Verification items for this drawing (mm, ordinates from the low corner). Round coordinates to 2 decimals unless told otherwise and drop trailing zeros. Order: outer loops, then holes, each group sorted by start corner. A loop starts at its lowest first (then second) coordinate and runs counter-clockwise, first axis right, second up. Notation, with made-up numbers: M -30.5,22.5 L -19.5,22.5 A12 ccw -19.5,30.5 Z; hole C 58.5,12.5 d5. An arc over 180 degrees is marked long. Use CSV: the item, a comma, the result in double quotes. Start each with the question number.
Q1. Sectioned sample at D-D (y = 6.5). Enter the section's corners in (x, z), and give its area (3 significant figures).
Q2. Scan lines: line 1 (Y direction, x = 20, z = 2.1); line 2 (Y direction, x = 20, z = 4.5); line 3 (X direction, y = 31.5, z = 0.9). Record each from-to range of solid material in increasing order.
Q3. Sectioned sample at C-C (z = 1.15). Enter the section's corners in (x, y).
Q4. Gauge pin test, flat ends, axial feed: pin 1 Ø0.9 at (x, y) = (45.5, 45) entering from +Z; pin 2 Ø2.5 at (x, y) = (20, 45) entering from +Z; pin 3 Ø3 at (x, z) = (29, 1.5) entering from +Y. Record the tip position at first contact, or that the pin passes through.
Q5. Sectioned sample at A-A (x = 45). Enter the section's corners in (y, z).
Q6. Sectioned sample at B-B (y = 45). Enter the section's corners in (x, z).
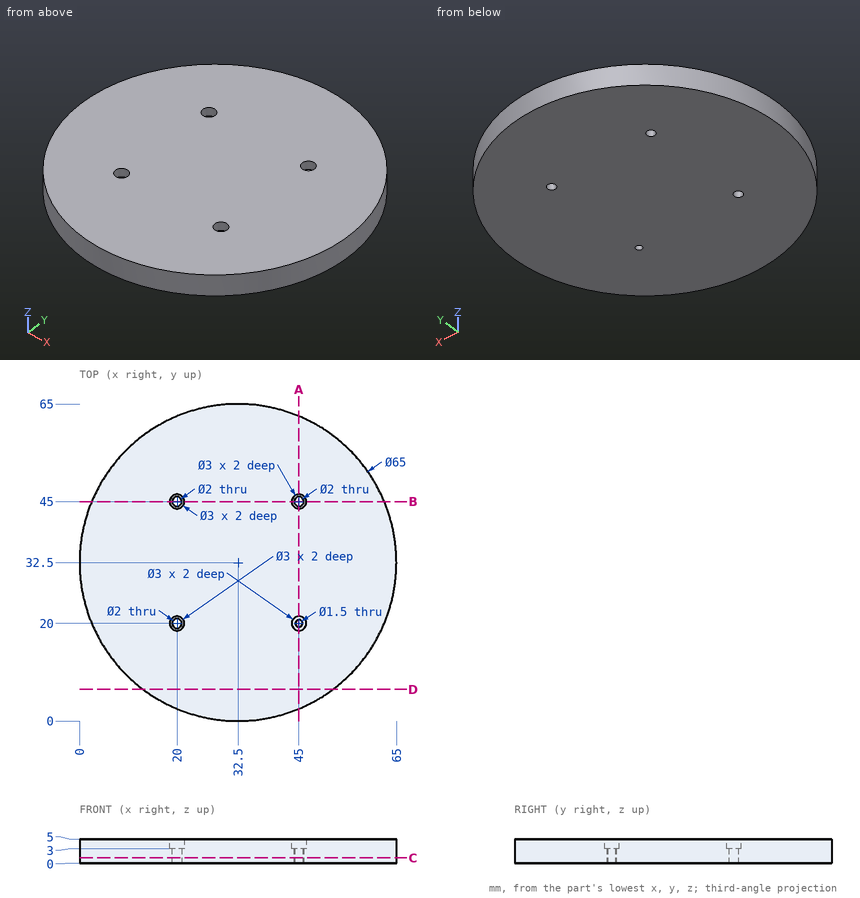
Verdict:
1,outline,"M 13,0 L 52,0 L 52,5 L 13,5 Z"
1,area,"195 mm²"
2,line 1,"y = 2.5 to 19, 21 to 44, 46 to 62.5"
2,line 2,"y = 2.5 to 18.5, 21.5 to 43.5, 46.5 to 62.5"
2,line 3,"x = 0.02 to 64.98"
3,outline,"C 32.5,32.5 d65; hole C 20,20 d2; hole C 20,45 d2; hole C 45,45 d2; hole C 45,20 d1.5"
4,pin 1,"passes through"
4,pin 2,"stops at z = 3"
4,pin 3,"stops at y = 64.94"
5,outline,"M 2.5,0 L 19.25,0 L 19.25,3 L 18.5,3 L 18.5,5 L 2.5,5 Z; M 20.75,0 L 44,0 L 44,3 L 43.5,3 L 43.5,5 L 21.5,5 L 21.5,3 L 20.75,3 Z; M 46,0 L 62.5,0 L 62.5,5 L 46.5,5 L 46.5,3 L 46,3 Z"
6,outline,"M 2.5,0 L 19,0 L 19,3 L 18.5,3 L 18.5,5 L 2.5,5 Z; M 21,0 L 44,0 L 44,3 L 43.5,3 L 43.5,5 L 21.5,5 L 21.5,3 L 21,3 Z; M 46,0 L 62.5,0 L 62.5,5 L 46.5,5 L 46.5,3 L 46,3 Z"
